The listing builds one solid part. Answer for the finished solid, in the listing's coordinates (mm). Face numbers are marked on the shaded views. A direction names the side the tool comes from. Round coordinates to 2 decimals unless told otherwise and drop trailing zeros. Write each loop counter-clockwise with the first axis right and the second up, starting at its lowest first coordinate (ties: lowest second). Pieces come first, ordered by that corner, then holes. Notation, with made-up numbers: (-33, 41.5) - (-11, 41.5) arc R31 ccw to (-11, 68.5) - close; hole circle Ø3 at (-24, -6.75). An arc over 180 degrees is marked (long way). Return JSON: item names as keys, results as strings. Group by question number.
from build123d import *

# Parameters (mm, degrees)
SKETCH1_W                   = 52
SKETCH1_H                   = 48
BASE_DEPTH                  = 1.04
SKETCH3_W                   = 19.05
SKETCH3_H                   = 27.35
ETHERNET_USB_LINKPP_DEPTH   = 31.1658
SKETCH4_W                   = 12.5476
SKETCH4_H                   = 5.7404
USB_PORTS_DEPTH             = 8.89
ETHERNET_PORT_DEPTH         = 11.4681
SKETCH6_W                   = 7.874
SKETCH6_H                   = 13.97
HEADPHONE_JACK_DEPTH        = 12.2428
SKETCH7_R                   = 2.9972
SKETCH7_R_2                 = 1.7653
HEADPHONE_JACK_CIRCLE_DEPTH = 3.9751
SKETCH8_W                   = 4.8895
SKETCH8_H                   = 7.6708
DC_POWER_DEPTH              = 3.302
SKETCH9_R                   = 1.25
DC_POWER_HOLE_DEPTH         = 5.842
SKETCH10_R                  = 0.4
DC_POWER_PIN_DEPTH          = 4.1656
SKETCH11_W                  = 2.4638
SKETCH11_H                  = 5.461
PWM_PIN_BASE_DEPTH          = 3.0988
SKETCH12_W                  = 0.635
SKETCH12_H                  = 0.635
PWM_PINS_DEPTH              = 6.0452
SKETCH13_W                  = 6.5278
SKETCH13_H                  = 7.5184
MICRO_HDMI_PORT_DEPTH       = 2.9718
SKETCH14_W                  = 7.5184
SKETCH14_H                  = 5.4102
MICRO_USB_PORT_DEPTH        = 2.54
HEADER_HOLE_REACH           = 82.266
SKETCH15_R                  = 0.8636
SKETCH16_R                  = 1.9939
STANDOFFS_1_DEPTH           = 4.4704
SKETCH17_R                  = 1.9939
SHORT_STANDOFF_DEPTH        = 1.9939
THREADS_IN_STANDOFFS_REACH  = 82.266
SKETCH19_R                  = 0.8636
SKETCH20_W                  = 12.1158
SKETCH20_H                  = 12.1158
CPU_DEPTH                   = 1.4732
UART_PLASTIC_DEPTH          = 5.7912
UART_HOLE_DEPTH             = 4.1656
SKETCH23_W                  = 11.5062
SKETCH23_H                  = 5.5372
MICROSD_DEPTH               = 3.302
SKETCH24_W                  = 13.6398
SKETCH24_H                  = 18.2118
EMMC_BOARD_DEPTH            = 1.778
SKETCH25_W                  = 12.319
SKETCH25_H                  = 16.1544
EMMC_CHIP_DEPTH             = 0.7874


with BuildPart() as part:
    # Sketch1 → Base (new body)
    with BuildSketch(Plane(origin=(0, 0, 0), x_dir=(1, 0, 0), z_dir=(0, 1, 0))):
        with Locations((26, 24)):
            Rectangle(SKETCH1_W, SKETCH1_H)
    extrude(amount=BASE_DEPTH)

    # Sketch3 → Ethernet-USB-LinkPP (add)
    with BuildSketch(Plane(origin=(0, 1.04, 0), x_dir=(1, 0, 0), z_dir=(0, 1, 0))):
        with Locations((11.5316, 8.0362)):
            Rectangle(SKETCH3_W, SKETCH3_H)
    extrude(amount=ETHERNET_USB_LINKPP_DEPTH)

    # Sketch4 → USB ports (cut)
    with BuildSketch(Plane.XY.offset(5.6388)):
        with Locations((11.5316, 5.0786)):
            Rectangle(SKETCH4_W, SKETCH4_H)
        with Locations((11.5316, 13.3844)):
            Rectangle(SKETCH4_W, SKETCH4_H)
    extrude(amount=-USB_PORTS_DEPTH, mode=Mode.SUBTRACT)

    # Sketch5 → Ethernet port (cut)
    with BuildSketch(Plane.XY.offset(5.6388)):
        Polygon((5.2578, 27.1893), (8.2296, 27.1893), (8.2296, 28.9419), (9.5758, 28.9419), (9.5758, 30.7961), (13.4874, 30.7961), (13.4874, 28.9419), (14.8336, 28.9419), (14.8336, 27.1893), (17.8054, 27.1893), (17.8054, 20.4837), (5.2578, 20.4837), align=None)
    extrude(amount=-ETHERNET_PORT_DEPTH, mode=Mode.SUBTRACT)

    # Sketch6 → Headphone jack (add)
    with BuildSketch(Plane(origin=(0, 1.04, 0), x_dir=(1, 0, 0), z_dir=(0, 1, 0))):
        with Locations((3.9116, 41.0404)):
            Rectangle(SKETCH6_W, SKETCH6_H)
    extrude(amount=HEADPHONE_JACK_DEPTH)

    # Sketch7 → Headphone jack circle (add)
    with BuildSketch(Plane(origin=(0, 0, -48), x_dir=(-1, 0, 0), z_dir=(0, 0, -1))):
        with Locations(Location((-4.8514, 7.9107, 0), (0, 0, 180))):
            Circle(SKETCH7_R)
        with Locations(Location((-4.8514, 7.9107, 0), (0, 0, 180))):
            Circle(SKETCH7_R_2, mode=Mode.SUBTRACT)
    extrude(amount=HEADPHONE_JACK_CIRCLE_DEPTH)

    # Sketch8 → DC power (add)
    with BuildSketch(Plane(origin=(0, 1.04, 0), x_dir=(1, 0, 0), z_dir=(0, 1, 0))):
        with Locations((16.09725, 44.19)):
            Rectangle(SKETCH8_W, SKETCH8_H)
    extrude(amount=DC_POWER_DEPTH)

    # Sketch9 → DC power hole (cut)
    with BuildSketch(Plane(origin=(0, 0, -48.0254), x_dir=(-1, 0, 0), z_dir=(0, 0, -1))):
        with Locations((-16.09725, 2.3154)):
            Circle(SKETCH9_R)
    extrude(amount=-DC_POWER_HOLE_DEPTH, mode=Mode.SUBTRACT)

    # Sketch10 → DC power pin (add)
    with BuildSketch(Plane(origin=(0, 0, -42.1834), x_dir=(-1, 0, 0), z_dir=(0, 0, -1))):
        with Locations((-16.09725, 2.3154)):
            Circle(SKETCH10_R)
    extrude(amount=DC_POWER_PIN_DEPTH)

    # Sketch11 → PWM pin base (add)
    with BuildSketch(Plane(origin=(0, 1.04, 0), x_dir=(1, 0, 0), z_dir=(0, 1, 0))):
        with Locations((20.9739, 45.2949)):
            Rectangle(SKETCH11_W, SKETCH11_H)
    extrude(amount=PWM_PIN_BASE_DEPTH)

    # Sketch12 → PWM pins (add)
    with BuildSketch(Plane(origin=(0, 4.1388, 0), x_dir=(1, 0, 0), z_dir=(0, 1, 0))):
        with Locations((20.9739, 43.92965)):
            Rectangle(SKETCH12_W, SKETCH12_H)
        with Locations((20.9739, 46.66015)):
            Rectangle(SKETCH12_W, SKETCH12_H)
    extrude(amount=PWM_PINS_DEPTH)

    # Sketch13 → Micro HDMI port (add)
    with BuildSketch(Plane(origin=(0, 1.04, 0), x_dir=(1, 0, 0), z_dir=(0, 1, 0))):
        with Locations((32.8357, 44.6472)):
            Rectangle(SKETCH13_W, SKETCH13_H)
    extrude(amount=MICRO_HDMI_PORT_DEPTH)

    # Sketch14 → Micro USB port (add)
    with BuildSketch(Plane(origin=(0, 1.04, 0), x_dir=(1, 0, 0), z_dir=(0, 1, 0))):
        with Locations((47.5296, 46.1839)):
            Rectangle(SKETCH14_W, SKETCH14_H)
    extrude(amount=MICRO_USB_PORT_DEPTH)

    # Sketch15 → Header hole (cut, up to next)
    with BuildSketch(Plane(origin=(0, 0, 0), x_dir=(-1, 0, 0), z_dir=(0, -1, 0)), mode=Mode.PRIVATE) as header_hole_sk1:
        with Locations(Location((-3, 30.1, 0), (0, 0, 90))):
            Circle(SKETCH15_R)
    header_hole_tool1 = extrude(header_hole_sk1.sketch, amount=-HEADER_HOLE_REACH, mode=Mode.PRIVATE) & part.part
    # Sketch15 → Header hole (cut, up to next)
    with BuildSketch(Plane(origin=(0, 0, 0), x_dir=(-1, 0, 0), z_dir=(0, -1, 0)), mode=Mode.PRIVATE) as header_hole_sk2:
        with Locations(Location((-49, 21.8012, 0), (0, 0, 90))):
            Circle(SKETCH15_R)
    header_hole_tool2 = extrude(header_hole_sk2.sketch, amount=-HEADER_HOLE_REACH, mode=Mode.PRIVATE) & part.part
    # Sketch15 → Header hole (cut, up to next)
    with BuildSketch(Plane(origin=(0, 0, 0), x_dir=(-1, 0, 0), z_dir=(0, -1, 0)), mode=Mode.PRIVATE) as header_hole_sk3:
        with Locations(Location((-40.8, 44.9012, 0), (0, 0, 90))):
            Circle(SKETCH15_R)
    header_hole_tool3 = extrude(header_hole_sk3.sketch, amount=-HEADER_HOLE_REACH, mode=Mode.PRIVATE) & part.part
    add(header_hole_tool1.solids().sort_by_distance((3, 0, -30.1))[0], mode=Mode.SUBTRACT)
    add(header_hole_tool2.solids().sort_by_distance((49, 0, -21.8012))[0], mode=Mode.SUBTRACT)
    add(header_hole_tool3.solids().sort_by_distance((40.8, 0, -44.9012))[0], mode=Mode.SUBTRACT)

    # Sketch16 → Standoffs 1 (add)
    with BuildSketch(Plane.XZ):
        with Locations(Location((49, -21.8012, 0), (0, 0, 270))):
            Circle(SKETCH16_R)
        with Locations(Location((3, -30.1, 0), (0, 0, 270))):
            Circle(SKETCH16_R)
    extrude(amount=STANDOFFS_1_DEPTH)

    # Sketch17 → Short standoff (add)
    with BuildSketch(Plane.XZ):
        with Locations(Location((40.8, -44.9012, 0), (0, 0, 270))):
            Circle(SKETCH17_R)
    extrude(amount=SHORT_STANDOFF_DEPTH)

    # Sketch19 → Threads in standoffs (cut, up to next)
    with BuildSketch(Plane.XZ, mode=Mode.PRIVATE) as threads_in_standoffs_sk1:
        with Locations(Location((40.8, -44.9012, 0), (0, 0, 270))):
            Circle(SKETCH19_R)
    threads_in_standoffs_tool1 = extrude(threads_in_standoffs_sk1.sketch, amount=THREADS_IN_STANDOFFS_REACH, mode=Mode.PRIVATE) & part.part
    # Sketch19 → Threads in standoffs (cut, up to next)
    with BuildSketch(Plane.XZ, mode=Mode.PRIVATE) as threads_in_standoffs_sk2:
        with Locations(Location((49, -21.8012, 0), (0, 0, 270))):
            Circle(SKETCH19_R)
    threads_in_standoffs_tool2 = extrude(threads_in_standoffs_sk2.sketch, amount=THREADS_IN_STANDOFFS_REACH, mode=Mode.PRIVATE) & part.part
    # Sketch19 → Threads in standoffs (cut, up to next)
    with BuildSketch(Plane.XZ, mode=Mode.PRIVATE) as threads_in_standoffs_sk3:
        with Locations(Location((3, -30.1, 0), (0, 0, 270))):
            Circle(SKETCH19_R)
    threads_in_standoffs_tool3 = extrude(threads_in_standoffs_sk3.sketch, amount=THREADS_IN_STANDOFFS_REACH, mode=Mode.PRIVATE) & part.part
    add(threads_in_standoffs_tool1.solids().sort_by_distance((40.8, 0, -44.9012))[0], mode=Mode.SUBTRACT)
    add(threads_in_standoffs_tool2.solids().sort_by_distance((49, 0, -21.8012))[0], mode=Mode.SUBTRACT)
    add(threads_in_standoffs_tool3.solids().sort_by_distance((3, 0, -30.1))[0], mode=Mode.SUBTRACT)

    # Sketch20 → CPU (add)
    with BuildSketch(Plane(origin=(0, 0, 0), x_dir=(-1, 0, 0), z_dir=(0, -1, 0))):
        with Locations((-37.8141, 31.1979)):
            Rectangle(SKETCH20_W, SKETCH20_H)
    extrude(amount=CPU_DEPTH)

    # Sketch21 → UART plastic (add)
    with BuildSketch(Plane(origin=(0, 1.04, 0), x_dir=(1, 0, 0), z_dir=(0, 1, 0))):
        Polygon((52.0254, 38.1254), (47.1994, 38.1254), (47.1994, 27.192440979), (48.636240979, 25.7556), (52.0254, 25.7556), align=None)
    extrude(amount=UART_PLASTIC_DEPTH)

    # Sketch22 → UART hole (cut)
    with BuildSketch(Plane(origin=(0, 6.8312, 0), x_dir=(1, 0, 0), z_dir=(0, 1, 0))):
        Polygon((51.365, 37.465), (49.134996369, 37.465), (47.8598, 36.189803631), (47.8598, 27.465987616), (48.909787616, 26.416), (51.365, 26.416), align=None)
    extrude(amount=-UART_HOLE_DEPTH, mode=Mode.SUBTRACT)

    # Sketch23 → MicroSD (add)
    with BuildSketch(Plane(origin=(0, 1.04, 0), x_dir=(1, 0, 0), z_dir=(0, 1, 0))):
        with Locations((44.8499, 12.6238)):
            Rectangle(SKETCH23_W, SKETCH23_H)
    extrude(amount=MICROSD_DEPTH)

    # Sketch24 → eMMC board (add)
    with BuildSketch(Plane(origin=(0, 1.04, 0), x_dir=(1, 0, 0), z_dir=(0, 1, 0))):
        with Locations((32.1437, 11.1252)):
            Rectangle(SKETCH24_W, SKETCH24_H)
    extrude(amount=EMMC_BOARD_DEPTH)

    # Sketch25 → eMMC chip (add)
    with BuildSketch(Plane(origin=(0, 2.818, 0), x_dir=(1, 0, 0), z_dir=(0, 1, 0))):
        with Locations((32.1437, 10.1219)):
            Rectangle(SKETCH25_W, SKETCH25_H)
    extrude(amount=EMMC_CHIP_DEPTH)


solid = part.part
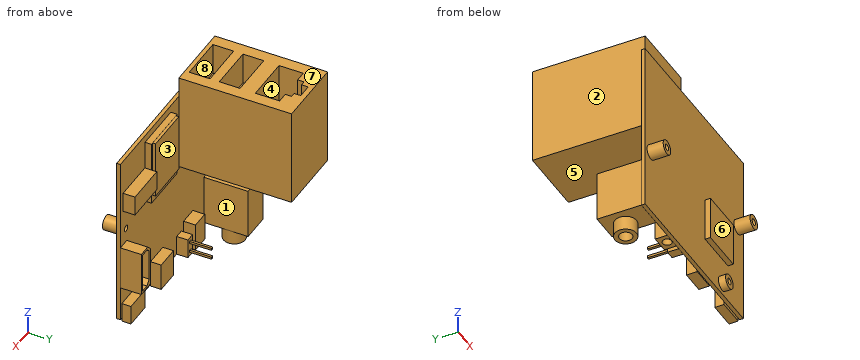
(1) Find section C-C (z = -30.1). Write down the section's boundary in (x, y) (3 decimals).
(2) Consider line 1 (X direction, y = -0.5, z = -30.1); line 2 (X direction, y = 15.5, z = 2.5); line 3 (X direction, y = 12, z = -41.5). Determine where each line is inside the solid, lowest interval first.
(3) Find section A-A (y = 12.5). Write down the section's boundary in (x, z).
(4) Find section D-D (z = -11). Write down the section's boundary in (x, y).
(5) For the marked faces 1, 2, 3, 4 and 5, determine the directions among +Z, -Z, +X, -X, +Y, -Y from which every point of the face is accessible in a straight line to the end or side of a thin tool.
(6) Flat-ended cylindrical pins translate along their axes: pin 1 (5 mm diameter, centred on x = 33, y = 0, fed in from -Z); pin 2 (0.9 mm diameter, centred on x = 33, y = 3.5, fed in from +Z); pin 3 (2 mm diameter, centred on x = 35, y = 2, fed in from +Z). Find the tip coordinate at first contact, or state that the pin passes through.
(7) Determine the mould class of the marked faces 6, 7 and 8 for opening direction Y: +Y half, -Y half, draft (parallel to the pull), parting line (faces both ways), or undercut.
(8) Find section B-B (x = 40.8). Write down the section's boundary in (y, z).
Check sheet entries:
{
 "1": {"outline": "(0, 0) - (1.006, 0) - (1.006, -4.47) - (2.136, -4.47) - (2.136, 1.04) - (0, 1.04) - close; (3.864, -4.47) - (4.994, -4.47) - (4.994, 0) - (31.756, 0) - (31.756, -1.473) - (43.872, -1.473) - (43.872, 0) - (52, 0) - (52, 1.04) - (52.025, 1.04) - (52.025, 6.831) - (51.365, 6.831) - (51.365, 2.666) - (47.86, 2.666) - (47.86, 6.831) - (47.199, 6.831) - (47.199, 1.04) - (3.864, 1.04) - close"},
 "2": {"line 1": "x = 1.01 to 2.14, 3.86 to 4.99, 31.76 to 43.87", "line 2": "x = 2.01 to 5.26, 17.81 to 21.06", "line 3": "x = -0.03 to 7.85"},
 "3": {"outline": "(-0.03, -48.03) - (7.85, -48.03) - (7.85, -34.06) - (-0.03, -34.06) - close; (2.01, -21.71) - (21.06, -21.71) - (21.06, 5.64) - (17.81, 5.64) - (17.81, -3.25) - (5.26, -3.25) - (5.26, 5.64) - (2.01, 5.64) - close"},
 "4": {"outline": "(0, 0) - (52, 0) - (52, 1.04) - (50.6, 1.04) - (50.6, 4.34) - (39.1, 4.34) - (39.1, 1.04) - (38.96, 1.04) - (38.96, 2.82) - (38.3, 2.82) - (38.3, 3.61) - (25.98, 3.61) - (25.98, 2.82) - (25.32, 2.82) - (25.32, 1.04) - (21.06, 1.04) - (21.06, 32.21) - (2.01, 32.21) - (2.01, 1.04) - (0, 1.04) - close"},
 "5": {"face 1": "-Z, +Y", "face 2": "+Z, -X, +Y", "face 3": "+Z, +Y", "face 4": "+Z", "face 5": "+X, -X, +Y"},
 "6": {"pin 1": "stops at z = -48.41", "pin 2": "stops at z = -2.04", "pin 3": "stops at z = 0"},
 "7": {"face 6": "-Y half", "face 7": "draft", "face 8": "undercut"},
 "8": {"outline": "(-1.99, -46.9) - (0, -46.9) - (0, -48) - (1.04, -48) - (1.04, -45.76) - (-1.99, -45.76) - close; (-1.99, -44.04) - (1.04, -44.04) - (1.04, -15.39) - (4.34, -15.39) - (4.34, -9.86) - (1.04, -9.86) - (1.04, 0) - (0, 0) - (0, -25.14) - (-1.47, -25.14) - (-1.47, -37.26) - (0, -37.26) - (0, -42.91) - (-1.99, -42.91) - close"}
}
